from build123d import *

# Parameters (mm, degrees)
BOSS_EXTRUDE1_DEPTH = 25
FILLET1_R           = 15
BOSS_EXTRUDE2_REACH = 69.823
SKETCH3_R           = 12.5
CUT_EXTRUDE1_DEPTH  = 68.823299831


with BuildPart() as part:
    # Sketch1 → Boss-Extrude1 (new, symmetric)
    with BuildSketch(Plane.XY):
        Polygon((60, 0), (70, 0), (70, 20), (0, 20), (0, 5), (60, 5), align=None)
    extrude(amount=BOSS_EXTRUDE1_DEPTH, both=True)

    # Fillet1
    fillet1_edges = [part.edges().sort_by_distance(p)[0] for p in [
        (0, 12.5, 25),
        (0, 12.5, -25),
    ]]
    fillet(fillet1_edges, radius=FILLET1_R)

    # Boss-Extrude2: up to this face of the body (flat: up to its plane)
    boss_extrude2_end = Plane(part.part.faces().sort_by_distance((35.898040292, 20, 0))[0])
    # Sketch2 → Boss-Extrude2 (add, up to the picked face)
    with BuildSketch(Plane(origin=(26.160254038, 45.310889132, 0), x_dir=(0, 0, -1), z_dir=(0.500000000000001, 0.866025403784438, 0)), mode=Mode.PRIVATE) as boss_extrude2_sk1:
        with BuildLine():
            Line((-20, -50.621778265), (20, -50.621778265))
            Line((20, -50.621778265), (20, -17.011053667))
            ThreePointArc((20, -17.011053667), (0, 2.988946333), (-20, -17.011053667))
            Line((-20, -17.011053667), (-20, -50.621778265))
        make_face()
    boss_extrude2_tool1 = split(extrude(boss_extrude2_sk1.sketch, amount=-BOSS_EXTRUDE2_REACH, mode=Mode.PRIVATE), bisect_by=boss_extrude2_end, keep=Keep.BOTH, mode=Mode.PRIVATE)
    add(boss_extrude2_tool1.solids().sort_by(Axis((48.469429, 32.430681, 0), (-0.500000000000001, -0.866025403784438, 0)))[0])

    # Sketch3 → Cut-Extrude1 (cut, through all)
    with BuildSketch(Plane(origin=(26.160254038, 45.310889132, 0), x_dir=(0, 0, -1), z_dir=(0.500000000000001, 0.866025403784438, 0))):
        with Locations(Location((0, -17.011053667, 0), (0, 0, 90))):
            Circle(SKETCH3_R)
    extrude(amount=-CUT_EXTRUDE1_DEPTH, mode=Mode.SUBTRACT)


solid = part.part
Could you check a few things on this model? Use its own coordinates, in mm. A direction names the side the tool comes from. Coordinates: 2 decimals unless noted, no trailing zeros. Loops run counter-clockwise (first coordinate to the right, second up) from the corner with the lowest first, then second, coordinate; pieces in that order, holes last.
1. I need wall thicknesses on L1, parallel to X at y = 28.5, z = 4.5; L2, parallel to X at y = 18, z = -5; L3, parallel to Z at x = 46.5, y = 28.5. Which ranges of each line are inside material? Lowest first, please.
2. For P1, Ø3, axis at x = 34.5, z = -13, coming from the +Y side; P2, Ø13.5, axis at x = 59.5, y = 26.5, coming from the -Z side; P3, Ø1, axis at y = 30.5, z = 3, coming from the +X side; P4, Ø2.5, axis at y = 3.5, z = -3.5, coming from the -X side, each with a flat end and sliding along its axis, tell me the tip position at first contact or that it passes through.
3. Imagine slicing it at C-C (x = 65). Please give me the cut outline in (y, z).
4. Imagine slicing it at B-B (z = -16). Please give me the cut outline in (x, y).
5. For faces 1 (the face through (48, 24, 20)), 2 (the face through (70, 10, 0)), 3 (the face through (60, 3, 0)), which set-ups out of +Z, -Z, +X, -X, +Y, -Y let a thin tool reach every point of the face, with its end or its side?
6. Imagine slicing it at D-D (z = 1). Please give me the cut outline in (x, y), and give its area (3 significant figures).
7. Imagine slicing it at A-A (z = -7). Please give me the cut outline in (x, y), and give its area (3 significant figures).
8. We'd pull the mould along Z, two halves only. Please class faces 4 (the face through (22.176, 28.234, 3.755)), 5 (the face through (47, 27, -20)), 6 (the face through (4.28, 12.4, 20.49)), 7 (the face through (22, 20, 19)): released by +Z, released by -Z, zero draft, split by the parting line, or undercut.
Computed values:
1. L1: x = 13.6 to 22.63, 49.56 to 55.28
1. L2: x = 0 to 16.81, 43.26 to 70
1. L3: z = -20 to -8.67, 8.67 to 20
2. P1: stops at y = 41.36
2. P2: stops at z = -25
2. P3: stops at x = 52.68
2. P4: stops at x = 60
3. outline: (0, -25) - (20, -25) - (20, -20) - (22.89, -20) - (22.89, 20) - (20, 20) - (20, 25) - (0, 25) - close
4. outline: (1.25, 5) - (60, 5) - (60, 0) - (70, 0) - (70, 20) - (30.5, 42.81) - (17.33, 20) - (1.25, 20) - close
5. face 1: +Z, +X, -X, +Y
5. face 2: +Z, -Z, +X, +Y, -Y
5. face 3: +Z, -Z, -X, -Y
6. outline: (0, 5) - (8.14, 5) - (30.1, 43.04) - (23.59, 46.79) - (8.12, 20) - (0, 20) - close; (36.92, 5) - (60, 5) - (60, 0) - (70, 0) - (70, 20) - (51.68, 30.58) - close
6. area: 1,010 mm2
7. outline: (0, 5) - (10.57, 5) - (31.92, 41.98) - (24.67, 46.17) - (9.56, 20) - (0, 20) - close; (34.49, 5) - (60, 5) - (60, 0) - (70, 0) - (70, 20) - (49.86, 31.63) - close
7. area: 1,130 mm2
8. face 4: undercut
8. face 5: released by -Z
8. face 6: released by +Z
8. face 7: zero draft
